Verification items for this drawing (mm, ordinates from the low corner). A direction names the side the tool comes from. Give positions to 0.01 mm unless a question says otherwise; leave off trailing zeros. Loops run counter-clockwise (first coordinate to the right, second up) from the corner with the lowest first, then second, coordinate; pieces in that order, holes last. Notation, with made-up numbers: (-8, 70) -> (22, 70) arc R23 cw to (22, 102) -> close; hole circle Ø9 at (38, 0.5). An arc over 180 degrees is marked (long way). Answer in a Markdown table with one row per item. Add a question column.
Q1. Set-up check for the marked faces 4, 5, 6, 7 and 8: record each of +Z, -Z, +X, -X, +Y, -Y from which the full face is reachable in a straight line by a thin tool's end or side.
Q2. Section check A-A on x = 1.85. Give the number of separate pieces and of enclosed holes in the cut face, and give its area (3 significant figures).
Q3. Material ranges on probe 1 along Y at (x, z) = (2.1, 22.5); probe 2 along Y at (x, z) = (0.25, 39.5); probe 3 along Z at (x, y) = (0.8, 14), recorded low to high.
Q4. Gauge pin test, flat ends, axial feed: P1, Ø19, axis at y = 17.78, z = 22.225, coming from the -X side; P2, Ø2.5, axis at x = 3, z = 43, coming from the -Y side; P3, Ø1.5, axis at x = 1.5, y = 2, coming from the +Z side; P4, Ø2.5, axis at x = 2, y = 2, coming from the -Z side. Record the tip position at first contact, or that the pin passes through.
Q5. Section check D-D on y = 25. Enter the section's corners in (x, z), and give its area (3 significant figures).
Q6. Release check for a two-part mould opening along Z. For the marked faces 1, 2 and 3 record: pulls with the +Z half, pulls with the -Z half, needs draft (parallel to the pull), parting line crosses it, or undercut.
Q7. Section check C-C on z = 20.5. Enter the section's corners in (x, y).
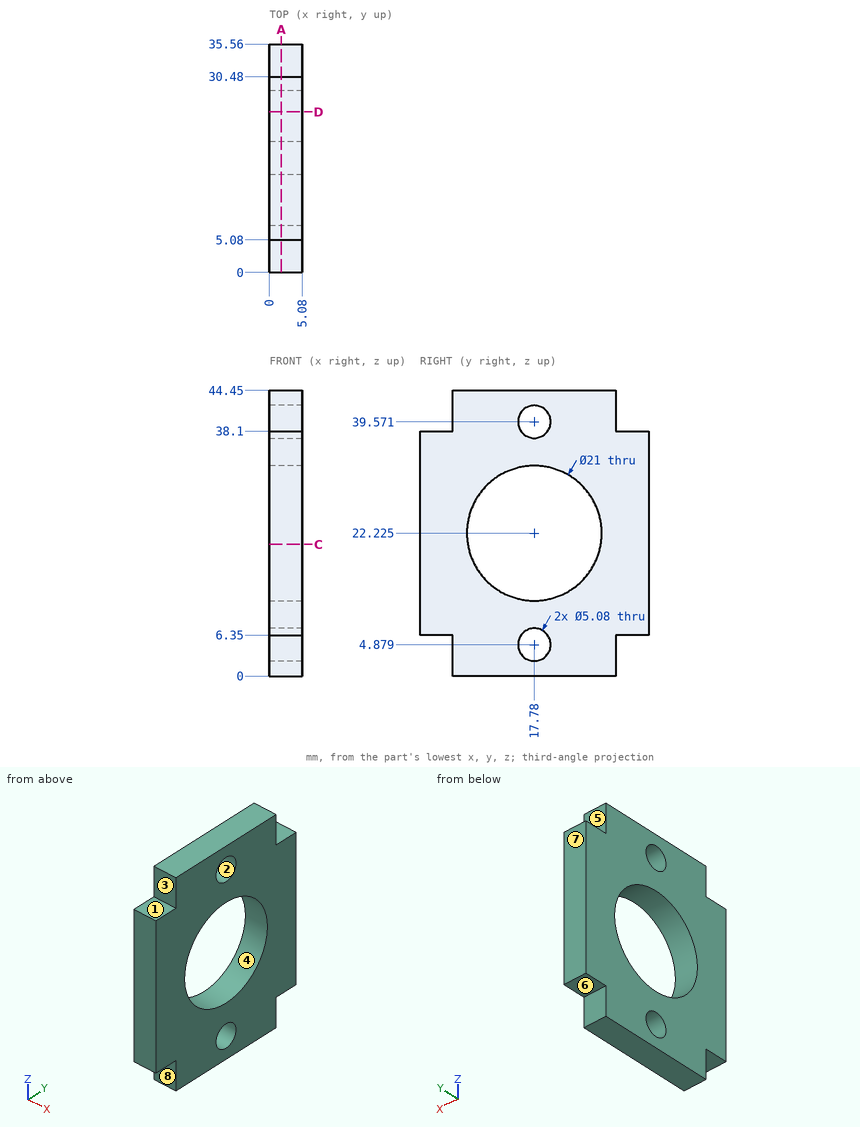
Taken from the geometry:
| question | item | result |
|---|---|---|
| 1 | face 4 | +X, -X |
| 1 | face 5 | +Z, +X, -X, +Y |
| 1 | face 6 | -Z, +X, -X, +Y |
| 1 | face 7 | +Z, -Z, +X, -X, +Y |
| 1 | face 8 | -Z, +X, -X, -Y |
| 2 | separate pieces | 1 |
| 2 | enclosed holes | 3 |
| 2 | area | 1,060 mm² |
| 3 | probe 1 | y = 0 to 7.28, 28.28 to 35.56 |
| 3 | probe 2 | y = 5.08 to 15.24, 20.32 to 30.48 |
| 3 | probe 3 | z = 0 to 12.43, 32.02 to 44.45 |
| 4 | P1 | passes through |
| 4 | P2 | stops at y = 5.08 |
| 4 | P3 | stops at z = 38.1 |
| 4 | P4 | stops at z = 6.35 |
| 5 | outline | (0, 0) -> (5.08, 0) -> (5.08, 14.6) -> (0, 14.6) -> close; (0, 29.85) -> (5.08, 29.85) -> (5.08, 44.45) -> (0, 44.45) -> close |
| 5 | area | 148 mm² |
| 6 | face 1 | pulls with the +Z half |
| 6 | face 2 | undercut |
| 6 | face 3 | needs draft |
| 7 | outline | (0, 0) -> (5.08, 0) -> (5.08, 7.42) -> (0, 7.42) -> close; (0, 28.14) -> (5.08, 28.14) -> (5.08, 35.56) -> (0, 35.56) -> close |
